Here's how the part is built. I have some questions about the finished solid (model axes, mm). Face numbers are marked on the shaded views. A direction names the side the tool comes from. Round coordinates to 2 decimals unless told otherwise and drop trailing zeros. Write each loop counter-clockwise with the first axis right and the second up, starting at its lowest first coordinate (ties: lowest second). Pieces come first, ordered by that corner, then holes. Notation, with made-up numbers: M 8.25,57.25 L 37.25,57.25 A22 ccw 37.25,83.25 Z; hole C 13.5,26.25 d9. An arc over 180 degrees is marked long. Write item = value, one per line. Start each with the question number.
(1) On a 3-axis mill with a long thin cutter (end or side, diameter ignored), from which of +Z, -Z, +X, -X, +Y, -Y can I reach the whole of each face in a straight line? I mean the marked faces 3 and 4. Say none if no direction works.
(2) I need wall thicknesses on line 1 along Y through (x, z) = (4.75, 5); line 2 along Z through (x, y) = (9, 1.2). Which ranges of each line are inside material? Lowest first, please.
(3) I want a section at B-B (x = 8.5). List the corners of the cut face in (y, z) for me.
(4) Will these pins go through, and if not, where does the flat tip stop? pin 1 Ø1.6 at (y, z) = (1.5, -9) entering from +X; pin 2 Ø1.6 at (y, z) = (1.5, -8.5) entering from -X; pin 3 Ø1.2 at (x, y) = (8, 1.5) entering from +Z.
(5) I want a section at C-C (z = -5.25). List the corners of the cut face in (x, y) for me.
(6) I want a section at A-A (y = 1.7). List the corners of the cut face in (x, z) for me, and give its area (3 significant figures).
(7) If we mould it in two halves opening along X, with no side actions, what happens to the marked faces 1 and 2? For each: released by +X, released by -X, zero draft, split by the parting line, or undercut.
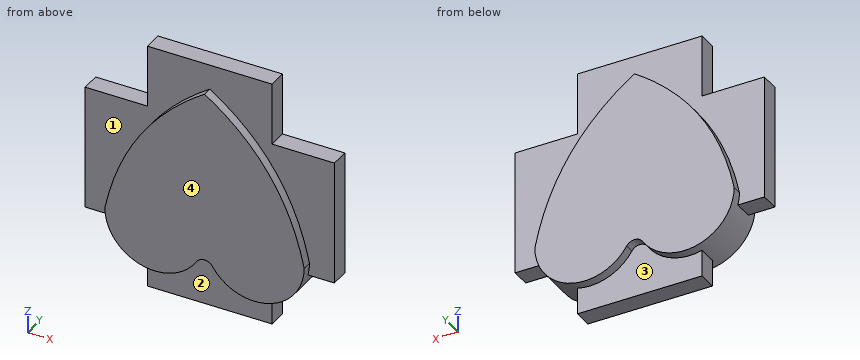
```python
from build123d import *

# Parameters (mm, degrees)
BOSS_EXTRUDE3_DEPTH      = 3
SKETCH2_W                = 8.5
SKETCH2_H                = 10
SKETCH2_W_2              = 10
SKETCH2_H_2              = 20
BOSS_EXTRUDE4_DEPTH      = 0.75
BOSS_EXTRUDE4_DEPTH_BACK = 0.75


with BuildPart() as part:
    # Sketch1 → Boss-Extrude3 (new body)
    with BuildSketch(Plane(origin=(0, 0, 0), x_dir=(1, 0, 0), z_dir=(0, 1, 0))):
        with BuildLine():
            ThreePointArc((-0.631578947, 6.157252793), (-5.123902974, 7.83885948), (-8, 4))
            add(Edge.make_bspline(
                [(-8, 4), (-6.403336947, -3.811544104), (0, -8)],
                knots=[0, 0, 0, 1, 1, 1], degree=2))
            add(Edge.make_bspline(
                [(8, 4), (6.403336947, -3.811544104), (0, -8)],
                knots=[0, 0, 0, 1, 1, 1], degree=2))
            ThreePointArc((8, 4), (5.123902974, 7.83885948), (0.631578947, 6.157252793))
            ThreePointArc((0.631578947, 6.157252793), (0, 5.811737691), (-0.631578947, 6.157252793))
        make_face()
    extrude(amount=BOSS_EXTRUDE3_DEPTH)

    # Sketch2 → Boss-Extrude4 (add, two sides)
    with BuildSketch(Plane(origin=(0, 1.5, 0), x_dir=(1, 0, 0), z_dir=(0, 1, 0))) as boss_extrude4_sk:
        with Locations((-5.75, 0)):
            Rectangle(SKETCH2_W, SKETCH2_H)
        with Locations((5.75, 0)):
            Rectangle(SKETCH2_W, SKETCH2_H)
        Rectangle(SKETCH2_W_2, SKETCH2_H_2)
        with BuildLine():
            ThreePointArc((8, 3.999999998), (5.123902975, 7.838859479), (0.631578947, 6.157252793))
            ThreePointArc((0.631578947, 6.157252793), (0, 5.811737691), (-0.631578947, 6.157252793))
            ThreePointArc((-0.631578947, 6.157252793), (-5.123902974, 7.83885948), (-8, 4))
            add(Edge.make_bspline(
                [(-8, 4), (-6.403336946, -3.811544103), (3e-09, -7.999999998)],
                knots=[0, 0, 0, 1, 1, 1], degree=2))
            add(Edge.make_bspline(
                [(3e-09, -7.999999998), (6.403336946, -3.811544103), (8, 3.999999998)],
                knots=[0, 0, 0, 1, 1, 1], degree=2))
        make_face()
    extrude(amount=BOSS_EXTRUDE4_DEPTH)
    extrude(boss_extrude4_sk.sketch, amount=-BOSS_EXTRUDE4_DEPTH_BACK)


solid = part.part
```
Returned:
q1.face_3 = -Z, +Y
q1.face_4 = +Z, -Z, +X, -X, -Y
q2.line_1 = 0.75 to 2.25
q2.line_2 = -5 to 5
q3.outline = M 0.75,-5 L 2.25,-5 L 2.25,5 L 0.75,5 Z
q4.pin_1 = 5
q4.pin_2 = -5.52
q4.pin_3 = 5
q5.outline = M -7.8,0 L 7.8,0 L 7.8,3 L -7.8,3 Z
q6.outline = M -10,-5 L -7.87,-5 A4 ccw -5,-7.87 L -5,-10 L 5,-10 L 5,-7.87 A4 ccw 7.87,-5 L 10,-5 L 10,5 L 5,5 L 5,10 L -5,10 L -5,5 L -10,5 Z
q6.area = 311 mm²
q7.face_1 = zero draft
q7.face_2 = undercut
